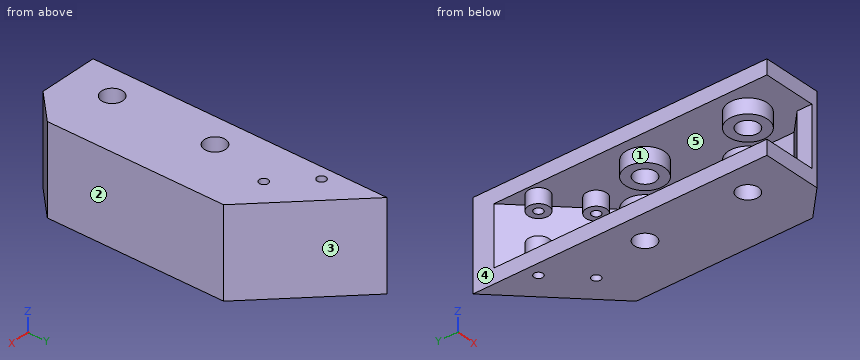
Autodesk Inventor part; units mm, degrees
ref_plane "Work Plane1" through (0, 0, 15) normal (0, 0, 1) x (1, 0, 0)
ref_plane "YZ Plane" through (0, 0, 0) normal (1, 0, 0) x (0, 1, 0)
ref_plane "XZ Plane" through (0, 0, 0) normal (0, 1, 0) x (-1, 0, 0)
sketch "Sketch3" plane through (0, 0, 0) normal (0, 0, 1) x (1, 0, 0)
  line L0 (0, 0) -> (0, 100)
  line L1 (0, 0) -> (20, 0)
  line L2 (20, 0) -> (30, 10)
  line L3 (30, 10) -> (30, 70)
  line L4 (30, 70) -> (0, 100)
  circle A0 centre (10, 15) radius 3.6
  circle A1 centre (10, 50) radius 3.6
  point P0 (10, 0)
  dimension "d6" = 100
  dimension "d7" = 20
  dimension "d13" = 10
  dimension "d14" = 10
  dimension "d15" = 7.2
  dimension "d16" = 7.2
  dimension "d17" = 35
  dimension "d18" = 15
  dimension "d33" = 135
extrude "Extrusion1" add sketch "Sketch3" along normal blind 30
ref_plane "Work Plane1" through (0, 0, 15) normal (0, 0, 1) x (1, 0, 0)
sketch "Sketch4" plane through (0, 0, 15) normal (0, 0, 1) x (1, 0, 0)
  line L0 (0, 100) -> (30, 70)
  line L1 (30, 70) -> (30, 10)
  line L2 (30, 10) -> (20, 0)
  line L3 (20, 0) -> (0, 0)
  line L4 (0, 92.9289) -> (25, 67.9289)
  line L5 (25, 67.9289) -> (25, 12.0711)
  line L6 (25, 12.0711) -> (17.9289, 5)
  line L7 (0, 0) -> (0, 100)
  line L8 (0, 5) -> (0, 92.9289)
  line L9 (17.9289, 5) -> (17.9289, 0)
  line L10 (17.9289, 0) -> (0, 0)
  line L11 (0, 5) -> (0, 0)
  dimension "d21" = 5
extrude "Extrusion2" cut sketch "Sketch4" along normal mid plane 20 contours L4 L5 L6 L9 L3 L7
sketch "Sketch5" plane through (0, 0, 30) normal (0, 0, 1) x (1, 0, 0)
  circle A0 centre (4.3934, 81.4645) radius 1.5
  circle A1 centre (15, 70.8579) radius 1.5
  line L0 (30, 70) -> (0, 100) construction
  line L1 (4.3934, 81.4645) -> (5.8076, 80.0503) construction
  line L2 (5.8076, 80.0503) -> (12.8787, 87.1213) construction
  line L3 (5.8076, 80.0503) -> (15, 70.8579) construction
  point P0 (0, 0)
  point P1 (15, 85)
  dimension "d24" = 3
  dimension "d25" = 3
  dimension "d35" = 2
  dimension "d37" = 13
  dimension "d38" = 10
extrude "Extrusion3" cut sketch "Sketch5" against normal through all
sketch "Sketch7" plane through (0, 0, 5) normal (0, 0, 1) x (1, 0, 0)
  circle A0 centre (10, 50) radius 3.6
  circle A1 centre (10, 15) radius 3.6
  circle A2 centre (10, 50) radius 6.6
  circle A3 centre (10, 15) radius 6.6
  point P0 (0, 0)
  dimension "d45" = 3
  dimension "d46" = 3
extrude "Extrusion5" add sketch "Sketch7" along normal blind 5
sketch "Sketch8" plane through (0, 0, 25) normal (0, 0, -1) x (-1, 0, 0)
  circle A0 centre (-10, 50) radius 3.6
  circle A1 centre (-10, 15) radius 3.6
  circle A2 centre (-10, 50) radius 6.6
  circle A3 centre (-10, 15) radius 6.6
  point P0 (0, 0)
  dimension "d49" = 3
  dimension "d50" = 3
extrude "Extrusion6" add sketch "Sketch8" along normal blind 5
sketch "Sketch9" plane through (0, 0, 5) normal (0, 0, 1) x (1, 0, 0)
  circle A0 centre (4.3934, 81.4645) radius 1.5
  circle A1 centre (15, 70.8579) radius 1.5
  circle A2 centre (4.3934, 81.4645) radius 3.5
  circle A3 centre (15, 70.8579) radius 3.5
  point P0 (0, 0)
  dimension "d53" = 2
  dimension "d54" = 2
extrude "Extrusion7" add sketch "Sketch9" along normal blind 5
sketch "Sketch10" plane through (0, 0, 25) normal (0, 0, -1) x (-1, 0, 0)
  circle A0 centre (-4.3934, 81.4645) radius 1.5
  circle A1 centre (-15, 70.8579) radius 1.5
  circle A2 centre (-4.3934, 81.4645) radius 3.5
  circle A3 centre (-15, 70.8579) radius 3.5
  point P0 (0, 0)
  dimension "d57" = 2
  dimension "d58" = 2
extrude "Extrusion8" add sketch "Sketch10" along normal blind 5
properties part number "GA005" material "ABS Plastic"
Verification items for the finished model (mm, model axes). Face numbers are marked on the shaded views. A direction names the side the tool comes from. Round coordinates to 2 decimals unless told otherwise and drop trailing zeros. Write each loop counter-clockwise with the first axis right and the second up, starting at its lowest first coordinate (ties: lowest second). Pieces come first, ordered by that corner, then holes. Notation, with made-up numbers: (38, 55) -> (72, 55) arc R16 ccw to (72, 83) -> close; hole circle Ø8 at (20.5, 5). An arc over 180 degrees is marked (long way). Write each question's results on one line, items separated by ' | '.
Q1. Sectioned sample at B-B, the plane z = 21.25. Give the number of separate pieces and of enclosed holes in the cut face, and give its area (3 significant figures).
Derived:
separate pieces: 5 | enclosed holes: 4 | area: 805 mm²
Q2. Draft check along Y on the marked faces 3, 4 and 5. Enter one of: released by +Y, released by -Y, zero draft, split by the parting line, or undercut.
Derived:
face 3: released by +Y | face 4: zero draft | face 5: undercut
Q3. Go/stop test with flat-tipped pins: pin 1 Ø1.8 at (x, y) = (4.39, 81.46) entering from +Z; pin 2 Ø10 at (x, z) = (21, 18) entering from +Y; pin 3 Ø8 at (y, z) = (46.5, 17) entering from -X; pin 4 Ø16 at (y, z) = (32.5, 14.5) entering from -X. Record where each tip stops, or that it passes through.
Derived:
pin 1: passes through | pin 2: stops at y = 84 | pin 3: stops at x = 3.46 | pin 4: stops at x = 25
Q4. Sectioned sample at C-C, the plane y = 33. Record the boundary of the cut face in (x, z), and give its area (3 significant figures).
Derived:
outline: (0, 0) -> (30, 0) -> (30, 30) -> (0, 30) -> (0, 25) -> (25, 25) -> (25, 5) -> (0, 5) -> close | area: 400 mm²
Q5. Thickness scan on probe 1 along Z at (x, y) = (4, 27.5); probe 2 along Y at (x, z) = (10, 27.35); probe 3 along Z at (x, y) = (4, 52.5). Record the ranges inside material, lowest first.
Derived:
probe 1: z = 0 to 5, 25 to 30 | probe 2: y = 0 to 11.4, 18.6 to 46.4, 53.6 to 90 | probe 3: z = 0 to 10, 20 to 30
Q6. Sectioned sample at A-A, the plane y = 50. Record the boundary of the cut face in (x, z).
Derived:
outline: (0, 0) -> (6.4, 0) -> (6.4, 10) -> (3.4, 10) -> (3.4, 5) -> (0, 5) -> close; (0, 25) -> (3.4, 25) -> (3.4, 20) -> (6.4, 20) -> (6.4, 30) -> (0, 30) -> close; (13.6, 0) -> (30, 0) -> (30, 30) -> (13.6, 30) -> (13.6, 20) -> (16.6, 20) -> (16.6, 25) -> (25, 25) -> (25, 5) -> (16.6, 5) -> (16.6, 10) -> (13.6, 10) -> close
Q7. Access from +Z, -Z, +X, -X, +Y, -Y to the whole of each face (thin tool, end or side, straight path). Record for the marked faces 1 and 2.
Derived:
face 1: none | face 2: +Z, -Z, +X, +Y, -Y
Q8. Sectioned sample at D-D, the plane z = 11.5. Record the boundary of the cut face in (x, y), and give its area (3 significant figures).
Derived:
outline: (0, 92.93) -> (25, 67.93) -> (25, 12.07) -> (17.93, 5) -> (17.93, 0) -> (20, 0) -> (30, 10) -> (30, 70) -> (0, 100) -> close | area: 550 mm²
